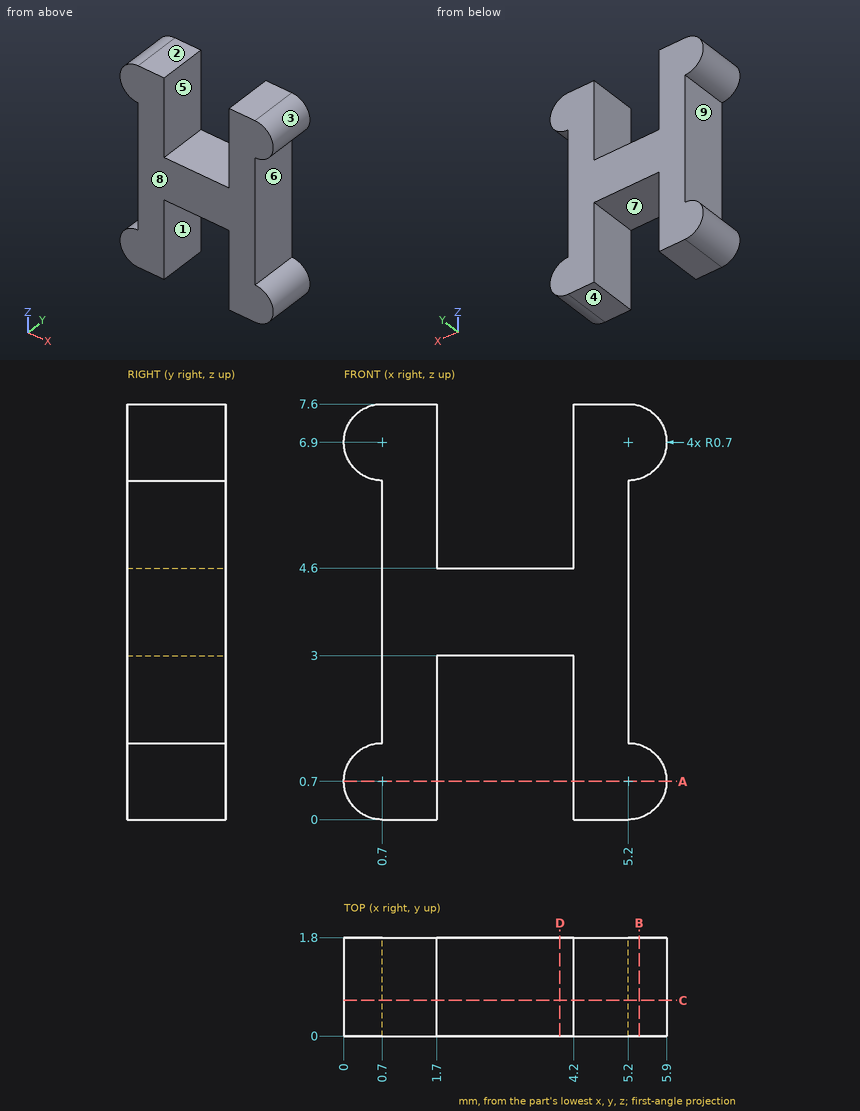
Input: dimensioned drawing with shaded views. Units: mm. Origin: part minimum x, y, z. A direction names the side the tool comes from. Coordinates: 2 decimals unless noted, no trailing zeros. Order: outer loops, then holes, each group sorted by start corner. A loop starts at its lowest first (then second) coordinate and runs counter-clockwise, first axis right, second up. Notation, with made-up numbers: M 87.25,22 L 102.25,22 A22 cw 102.25,46 Z; hole C 67.25,35.5 d10. An arc over 180 degrees is marked long. Answer as CSV lines item,"result".
Q1. Section D-D on x = 3.95. Return the cut outline in (y, z).
Answers:
outline,"M 0,3 L 1.8,3 L 1.8,4.6 L 0,4.6 Z"
Q2. Section B-B on x = 5.4. Return the cut outline in (y, z), and give its area (3 significant figures).
Answers:
outline,"M 0,0.03 L 1.8,0.03 L 1.8,1.37 L 0,1.37 Z; M 0,6.23 L 1.8,6.23 L 1.8,7.57 L 0,7.57 Z"
area,"4.83 mm^2"
Q3. Draft query along Z for the marked faces 1, 2, 3 and 4. Return one class per face: pulls with the +Z half, pulls with the -Z half, needs draft (parallel to the pull), parting line crosses it, or undercut.
Answers:
face 1,"needs draft"
face 2,"pulls with the +Z half"
face 3,"undercut"
face 4,"pulls with the -Z half"
Q4. Section A-A on z = 0.7. Return the cut outline in (x, y).
Answers:
outline,"M 0,0 L 1.7,0 L 1.7,1.8 L 0,1.8 Z; M 4.2,0 L 5.9,0 L 5.9,1.8 L 4.2,1.8 Z"
Q5. Set-up query: the marked faces 5, 6, 7, 8 and 9. Return all of +Z, -Z, +X, -X, +Y, -Y with unobstructed straight access to the full face (end or side cutting, diameter ignored); none if empty.
Answers:
face 5,"+Z, +Y, -Y"
face 6,"+X, +Y, -Y"
face 7,"-Z, +Y, -Y"
face 8,"+Z, -Z, +X, -X, -Y"
face 9,"-X, +Y, -Y"
Q6. First-contact query: P1, Ø0.9, axis at y = 1, z = 3.5, coming from the -X side; P2, Ø0.9, axis at x = 3.5, y = 1.5, coming from the -Z side; P3, Ø0.5, axis at x = 3.5, y = 0.5, coming from the +Z side. Flat tips, straight axial feed; report the tip coordinate or a pass-through.
Answers:
P1,"stops at x = 0.7"
P2,"stops at z = 3"
P3,"stops at z = 4.6"
Q7. Section C-C on y = 0.65. Return the cut outline in (x, z), and give its area (3 significant figures).
Answers:
outline,"M 0.7,0 L 1.7,0 L 1.7,3 L 4.2,3 L 4.2,0 L 5.2,0 A0.7 ccw 5.2,1.4 L 5.2,6.2 A0.7 ccw 5.2,7.6 L 4.2,7.6 L 4.2,4.6 L 1.7,4.6 L 1.7,7.6 L 0.7,7.6 A0.7 ccw 0.7,6.2 L 0.7,1.4 A0.7 ccw Z"
area,"22.3 mm^2"
Q8. Line query: probe 1 along X at (y, z) = (1.65, 2.25); probe 2 along Z at (x, y) = (5.25, 1.4); probe 3 along X at (y, z) = (1.65, 0.5). Output: solid intervals per line, ascending. Write a range as [from, to].
Answers:
probe 1,"x = [0.7, 1.7], [4.2, 5.2]"
probe 2,"z = [0, 1.4], [6.2, 7.6]"
probe 3,"x = [0.03, 1.7], [4.2, 5.87]"
